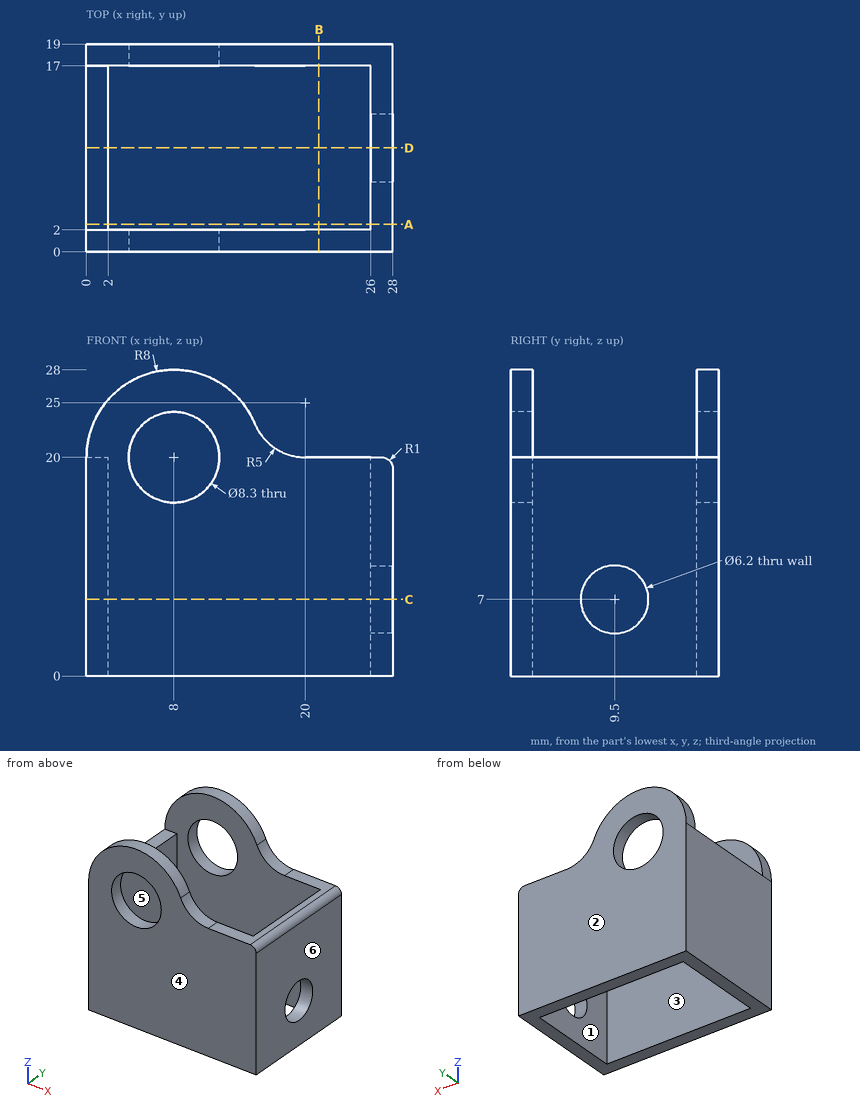
The drawing under review shows one solid part. Ordinate dimensions are in mm from its lowest x, y, z. A direction names the side the tool comes from. Coordinates: 2 decimals unless noted, no trailing zeros. Write each loop counter-clockwise with the first axis right and the second up, starting at its lowest first coordinate (ties: lowest second). Pieces come first, ordered by that corner, then holes.
1) Machinability: for the marked faces 1 and 2, which of the approach directions +Z, -Z, +X, -X, +Y, -Y give a long, thin tool a straight path to every point of the face, cutting with its end or side? Answer none if there is none.
2) Insertion check: pin 1 (7.5 mm diameter, centred on x = 22.5, y = 13, fed in from +Z); pin 2 (5.5 mm diameter, centred on y = 9.5, z = 7, fed in from +X). Each pin has a flat end and moves straight along its axis. Give the tip position at first contact, or say it passes through.
3) Add section C-C (z = 7). Write out the cut boundary in (x, y), plus the area to 3 significant figures.
4) Add section D-D (y = 9.5). Write out the cut boundary in (x, z).
5) To check wall thickness, follow L1, parallel to Z at x = 8, y = 1.1; L2, parallel to X at y = 5, z = 9; L3, parallel to Y at x = 27.6, z = 7. State the ranges of each line that lie inside material, in increasing order.
6) Mouldability with a two-part tool opening along Y and no side actions: class the marked faces 3, 4, 5 and 6 as +Y half, -Y half, draft (parallel to the pull), parting line (faces both ways), or undercut.
7) Add section B-B (x = 21.25). Write out the cut boundary in (y, z), plus the area to 3 significant figures.
8) Add section A-A (y = 2.5). Write out the cut boundary in (x, z).
Check result:
1. face 1: +Z, -Z
1. face 2: +Z, -Z, +X, -X, +Y
2. pin 1: stops at z = 20
2. pin 2: stops at x = 2
3. outline: (0, 0) - (28, 0) - (28, 6.4) - (26, 6.4) - (26, 2) - (2, 2) - (2, 17) - (26, 17) - (26, 12.6) - (28, 12.6) - (28, 19) - (0, 19) - close
3. area: 160 mm2
4. outline: (0, 0) - (2, 0) - (2, 20) - (0, 20) - close; (26, 0) - (28, 0) - (28, 3.9) - (26, 3.9) - close; (26, 10.1) - (28, 10.1) - (28, 19) arc R1 ccw to (27, 20) - (26, 20) - close
5. L1: z = 0 to 15.85, 24.15 to 28
5. L2: x = 0 to 2, 26 to 28
5. L3: y = 0 to 6.4, 12.6 to 19
6. face 3: undercut
6. face 4: -Y half
6. face 5: undercut
6. face 6: draft
7. outline: (0, 0) - (2, 0) - (2, 20) - (0, 20) - close; (17, 0) - (19, 0) - (19, 20) - (17, 20) - close
7. area: 80.0 mm2
8. outline: (0, 0) - (2, 0) - (2, 20) - (0, 20) - close; (26, 0) - (28, 0) - (28, 19) arc R1 ccw to (27, 20) - (26, 20) - close
